Autodesk Inventor part; units mm, degrees
ref_plane "YZ Plane" through (0, 0, 0) normal (1, 0, 0) x (0, 1, 0)
ref_plane "XZ Plane" through (0, 0, 0) normal (0, 1, 0) x (-1, 0, 0)
ref_plane "XY Plane" through (0, 0, 0) normal (0, 0, 1) x (1, 0, 0)
sketch "Sketch1" plane through (0, 0, 0) normal (0, 0, 1) x (1, 0, 0)
  line L0 (-65.0875, -53.975) -> (65.0875, -53.975)
  line L1 (65.0875, -53.975) -> (65.0875, 53.975)
  line L2 (65.0875, 53.975) -> (-65.0875, 53.975)
  line L3 (-65.0875, 53.975) -> (-65.0875, -53.975)
  line L4 (-65.0875, -53.975) -> (65.0875, 53.975) construction
  line L5 (65.0875, -53.975) -> (-65.0875, 53.975) construction
  point P0 (0, 0)
  dimension "d0" = 130.175
  dimension "d1" = 107.95
extrude "Extrusion1" add sketch "Sketch1" along normal blind 298.45
sketch "Sketch2" plane through (0, 0, 298.45) normal (0, 0, 1) x (1, 0, 0)
  line L0 (-65.0875, -53.975) -> (65.0875, -53.975) construction
  line L1 (-65.0875, 53.975) -> (-65.0875, -53.975) construction
  circle A0 centre (-23.8125, -22.225) radius 4
  circle A1 centre (23.8125, 9.525) radius 4
  line L2 (-11.1125, 12.065) -> (-33.3375, 12.065)
  line L3 (-33.3375, 12.065) -> (-33.3375, 13.335)
  line L4 (-33.3375, 13.335) -> (-11.1125, 13.335)
  line L5 (-11.1125, 13.335) -> (-11.1125, 12.065)
  line L6 (-33.3375, 12.7) -> (-65.0875, 12.7) construction
  point P0 (0, 0)
  dimension "d4" = 31.75
  dimension "d5" = 41.275
  dimension "d6" = 8
  dimension "d7" = 63.5
  dimension "d8" = 88.9
  dimension "d13" = 31.75
  dimension "d14" = 53.975
  dimension "d15" = 66.675
  dimension "d16" = 1.27
extrude "Extrusion2" add sketch "Sketch2" along normal blind 12.7
sketch "Sketch3" plane through (0, 0, 0) normal (0, 0, -1) x (-1, 0, 0)
  circle A0 centre (-23.8125, 9.525) radius 4
  circle A1 centre (23.8125, -22.225) radius 4
  line L0 (33.3375, 12.065) -> (11.1125, 12.065)
  line L1 (11.1125, 12.065) -> (11.1125, 13.335)
  line L2 (11.1125, 13.335) -> (33.3375, 13.335)
  line L3 (33.3375, 13.335) -> (33.3375, 12.065)
  point P0 (0, 0)
extrude "Extrusion3" add sketch "Sketch3" along normal blind 12.7
sketch "Sketch4" plane through (-33.3375, 13.335, 0) normal (0, 1, 0) x (1, 0, 0)
  line L0 (0, 12.7) -> (22.225, 12.7)
  line L1 (22.225, 0) -> (22.225, 12.7)
  line L2 (0, 0) -> (0, 12.7)
  line L3 (22.225, -298.45) -> (22.225, -311.15)
  line L4 (22.225, -311.15) -> (0, -311.15)
  line L5 (0, -298.45) -> (0, -311.15)
  line L6 (16.51, -308.61) -> (5.715, -308.61)
  line L7 (5.715, -308.61) -> (5.715, -304.165)
  line L8 (5.715, -304.165) -> (16.51, -304.165)
  line L9 (16.51, -304.165) -> (16.51, -308.61)
  line L10 (16.51, 5.715) -> (5.715, 5.715)
  line L11 (5.715, 5.715) -> (5.715, 10.16)
  line L12 (5.715, 10.16) -> (16.51, 10.16)
  line L13 (16.51, 10.16) -> (16.51, 5.715)
  line L14 (5.715, 10.16) -> (0, 12.7) construction
  line L15 (16.51, 10.16) -> (22.225, 12.7) construction
  line L16 (22.225, -311.15) -> (16.51, -308.61) construction
  line L17 (5.715, -308.61) -> (0, -311.15) construction
  point P0 (33.3375, 0)
  dimension "d17" = 10.795
  dimension "d18" = 6.985
  dimension "d19" = 2.54
extrude "Extrusion4" cut sketch "Sketch4" against normal up to surface (1.27 mm away)
fillet "Fillet1" radius 3.175 4 edges at (-33.3375, 12.7, -12.7) (-11.1125, 12.7, -12.7) (-33.3375, 12.7, 311.15) (-11.1125, 12.7, 311.15)
thread "Thread1"
thread "Thread2"
thread "Thread3"
thread "Thread4"
sketch "Sketch5" plane through (-65.0875, 53.975, 0) normal (0, 1, 0) x (1, 0, 0)
  line L0 (25.2364, -11.8087) -> (114.825, -11.8087) construction
  line L1 (114.825, -11.8087) -> (114.825, -199.7093) construction
  line L2 (114.825, -199.7093) -> (25.2364, -199.7093) construction
  line L3 (25.2364, -199.7093) -> (25.2364, -11.8087) construction
  line L4 (91.6181, -23.1502) -> (83.0142, -23.1502)
  line L5 (83.0142, -23.1502) -> (83.0142, -31.7541)
  line L6 (83.0142, -31.7541) -> (80.1737, -31.7541)
  line L7 (80.1737, -31.7541) -> (80.1737, -23.1502)
  line L8 (80.1737, -23.1502) -> (71.5698, -23.1502)
  line L9 (71.5698, -23.1502) -> (71.5698, -20.4126)
  line L10 (71.5698, -20.4126) -> (80.1737, -20.4126)
  line L11 (80.1737, -20.4126) -> (80.1737, -11.8087)
  line L12 (80.1737, -11.8087) -> (83.0142, -11.8087)
  line L13 (83.0142, -11.8087) -> (83.0142, -20.4126)
  line L14 (83.0142, -20.4126) -> (91.6181, -20.4126)
  line L15 (91.6181, -20.4126) -> (91.6181, -23.1502)
  line L16 (33.7374, -158.3681) -> (33.7374, -135.9732)
  line L17 (33.7374, -135.9732) -> (25.2158, -135.9732)
  line L18 (25.2158, -135.9732) -> (25.2158, -132.9681)
  line L19 (25.2158, -132.9681) -> (45.6346, -132.9681)
  line L20 (45.6346, -132.9681) -> (45.6346, -135.9732)
  line L21 (45.6346, -135.9732) -> (37.1131, -135.9732)
  line L22 (37.1131, -135.9732) -> (37.1131, -158.3681)
  line L23 (37.1131, -158.3681) -> (33.7374, -158.3681)
  spline S0 degree 2 poles (66.1769, -135.8703) (67.6178, -137.5582) (69.2233, -142.4982) (69.2233, -145.6681) knots 0 0 0 1 2 2 2
  spline S1 degree 2 poles (69.2233, -145.6681) (69.2233, -148.7556) (67.6589, -153.7574) (66.1769, -155.4452) knots 0 0 0 1 2 2 2
  spline S2 degree 2 poles (66.1769, -155.4452) (64.6126, -157.2154) (60.4753, -158.9032) (57.9847, -158.9032) knots 0 0 0 1 2 2 2
  spline S3 degree 2 poles (57.9847, -158.9032) (55.4118, -158.9032) (51.2951, -157.1536) (49.7925, -155.4452) knots 0 0 0 1 2 2 2
  spline S4 degree 2 poles (49.7925, -155.4452) (48.3311, -153.7574) (46.7667, -148.7967) (46.7667, -145.6681) knots 0 0 0 1 2 2 2
  spline S5 degree 2 poles (46.7667, -145.6681) (46.7667, -142.4776) (48.3516, -137.6199) (49.8131, -135.8703) knots 0 0 0 1 2 2 2
  spline S6 degree 2 poles (49.8131, -135.8703) (51.2951, -134.1825) (55.4324, -132.4329) (57.9847, -132.4329) knots 0 0 0 1 2 2 2
  spline S7 degree 2 poles (57.9847, -132.4329) (60.5782, -132.4329) (64.7361, -134.2442) (66.1769, -135.8703) knots 0 0 0 1 2 2 2
  spline S8 degree 2 poles (65.7035, -145.6681) (65.7035, -143.1569) (64.6126, -139.2666) (63.6246, -137.9904) knots 0 0 0 1 2 2 2
  spline S9 degree 2 poles (63.6246, -137.9904) (62.616, -136.6731) (59.7755, -135.3557) (58.0053, -135.3557) knots 0 0 0 1 2 2 2
  spline S10 degree 2 poles (58.0053, -135.3557) (56.1734, -135.3557) (53.4152, -136.6319) (52.3654, -137.9904) knots 0 0 0 1 2 2 2
  spline S11 degree 2 poles (52.3654, -137.9904) (51.3568, -139.2872) (50.2865, -143.198) (50.2865, -145.6681) knots 0 0 0 1 2 2 2
  spline S12 degree 2 poles (50.2865, -145.6681) (50.2865, -150.6698) (54.4855, -155.9804) (58.0053, -155.9804) knots 0 0 0 1 2 2 2
  spline S13 degree 2 poles (58.0053, -155.9804) (61.5251, -155.9804) (65.7035, -150.6698) (65.7035, -145.6681) knots 0 0 0 1 2 2 2
  spline S14 degree 2 poles (88.9834, -140.6251) (88.9834, -142.2718) (87.8102, -145.2358) (86.7604, -146.265) knots 0 0 0 1 2 2 2
  spline S15 degree 2 poles (86.7604, -146.265) (85.4431, -147.5617) (81.8821, -148.8997) (79.1651, -148.8997) knots 0 0 0 1 2 2 2
  line L24 (79.1651, -148.8997) -> (76.304, -148.8997)
  line L25 (76.304, -148.8997) -> (76.304, -158.3681)
  line L26 (76.304, -158.3681) -> (72.9283, -158.3681)
  line L27 (72.9283, -158.3681) -> (72.9283, -132.9681)
  line L28 (72.9283, -132.9681) -> (79.3092, -132.9681)
  spline S16 degree 2 poles (79.3092, -132.9681) (81.5734, -132.9681) (84.7432, -133.7091) (85.9576, -134.553) knots 0 0 0 1 2 2 2
  spline S17 degree 2 poles (85.9576, -134.553) (87.3779, -135.5204) (88.9834, -138.505) (88.9834, -140.6251) knots 0 0 0 1 2 2 2
  spline S18 degree 2 poles (85.4636, -140.728) (85.4636, -139.4107) (84.558, -137.4758) (83.6317, -136.8583) knots 0 0 0 1 2 2 2
  spline S19 degree 2 poles (83.6317, -136.8583) (82.829, -136.3232) (80.6883, -135.8909) (79.1034, -135.8909) knots 0 0 0 1 2 2 2
  line L29 (79.1034, -135.8909) -> (76.304, -135.8909)
  line L30 (76.304, -135.8909) -> (76.304, -146.018)
  line L31 (76.304, -146.018) -> (78.6093, -146.018)
  spline S20 degree 2 poles (78.6093, -146.018) (80.6677, -146.018) (83.1995, -145.3593) (84.0228, -144.4948) knots 0 0 0 1 2 2 2
  spline S21 degree 2 poles (84.0228, -144.4948) (84.7844, -143.7332) (85.4636, -141.9424) (85.4636, -140.728) knots 0 0 0 1 2 2 2
  line L32 (80.0296, -274.258) -> (70.4171, -274.258)
  line L33 (70.4171, -274.258) -> (70.4171, -271.1705)
  line L34 (70.4171, -271.1705) -> (80.0296, -271.1705)
  line L35 (80.0296, -271.1705) -> (80.0296, -274.258)
  point P0 (65.0875, 0)
extrude "Extrusion7" cut sketch "Sketch5" against normal blind 0.762
sketch "Sketch6" plane through (0, 0, 0) normal (0, 0, -1) x (-1, 0, 0)
  circle A0 centre (8.3375, 46.3906) radius 3.175
  point P0 (0, 0)
  dimension "d31" = 6.35
extrude "Extrusion5" add sketch "Sketch6" along normal blind 58.42
sketch "Sketch7" plane through (-8.3375, 46.3906, -58.42) normal (0, 0, -1) x (-1, 0, 0)
  circle A0 centre (0, 0) radius 3.175
  line L0 (-16.51, -7.3025) -> (16.51, -7.3025)
  line L1 (16.51, -7.3025) -> (16.51, 7.3025)
  line L2 (16.51, 7.3025) -> (-16.51, 7.3025)
  line L3 (-16.51, 7.3025) -> (-16.51, -7.3025)
  line L4 (-16.51, -7.3025) -> (16.51, 7.3025) construction
  line L5 (16.51, -7.3025) -> (-16.51, 7.3025) construction
  point P0 (-8.3375, -46.3906)
  dimension "d34" = 14.605
  dimension "d35" = 33.02
extrude "Extrusion6" add sketch "Sketch7" along normal blind 38.1 contours A0 | L3 L2 L1 L0
properties part number "12S Module"
The listing builds one solid part. Answer for the finished solid, in the listing's coordinates (mm). A direction names the side the tool comes from. Coordinates: 2 decimals unless noted, no trailing zeros. Loops run counter-clockwise (first coordinate to the right, second up) from the corner with the lowest first, then second, coordinate; pieces in that order, holes last. Notation, with made-up numbers: (32, 29) -> (89, 29) arc R35 cw to (89, 64) -> close; hole circle Ø3 at (27.5, 32.25). An arc over 180 degrees is marked (long way). Write item = value, one per line. Start each with the question number.
1) A cutting plane is placed at A-A (y = 0). Give the vertices of the cut face in (x, z), then the cut area to 3 significant figures.
2) A cutting plane is placed at B-B (x = 33). Give the vertices of the cut face in (y, z) (3 decimals), then the cut area to 3 significant figures.
3) Given pin 1 Ø12 at (x, y) = (-26.5, 16.5) entering from -Z; pin 2 Ø1.5 at (x, y) = (10, -7.5) entering from +Z; pin 3 Ø16 at (y, z) = (49, -86.5) entering from -X, each flat-ended and moving along its own axis, determine where each tip first touches the part or whether it passes through.
4) A tool of negligible diameter and unlimited length cuts with its end or side. For faces 4 (the face through (8.172, 46, -77)), 5 (the face through (-22, 12.065, -5)), 6 (the face through (26.987, 11.959, -6.261)), 7 (the face through (-24, -22, -12.7)), from which of +Z, -Z, +X, -X, +Y, -Y can it reach the whole face along a straight path? Write none if from no direction.
5) The mould has two halves that part along X. Classify faces 1 (the face through (-24, -22, 311.15)), 2 (the face through (-65.088, 1, 147)), 3 (the face through (-15, 53.213, 148)): released by +X, released by -X, zero draft, split by the parting line, or undercut.
6) Straight lines are drawn through the part: line 1 (Z direction, x = 13, y = -36.5); line 2 (Y direction, x = 11, z = 150) (3 decimals). For each, find the intervals that lie inside material, in ascending order. Write a range as from..to.
Responses:
q1.outline = (-65.09, 0) -> (65.09, 0) -> (65.09, 298.45) -> (-65.09, 298.45) -> close
q1.area = 38,900 mm²
q2.outline = (-53.975, 0) -> (53.975, 0) -> (53.975, 298.45) -> (-53.975, 298.45) -> close
q2.area = 32,200 mm²
q3.pin_1 = -12.7
q3.pin_2 = 298.45
q3.pin_3 = -24.85
q4.face_4 = -Z, +X, +Y, -Y
q4.face_5 = -Z, -X
q4.face_6 = -Z
q4.face_7 = -Z, +X, -X, +Y, -Y
q5.face_1 = zero draft
q5.face_2 = released by -X
q5.face_3 = undercut
q6.line_1 = 0..298.45
q6.line_2 = -53.975..53.213
